```python
from build123d import *

# Parameters (mm, degrees)
BOSS_EXTRUDE1_DEPTH = 160
CUT_EXTRUDE1_START  = -5
SKETCH2_R           = 5
SKETCH2_W           = 10
SKETCH2_H           = 16.92618617
CUT_EXTRUDE1_DEPTH  = 5
CUT_EXTRUDE2_START  = -160
SKETCH2_3_R         = 5
SKETCH2_3_W         = 16.92618617
SKETCH2_3_H         = 10
SKETCH2_3_W_2       = 10
SKETCH2_3_H_2       = 16.92618617
CUT_EXTRUDE2_DEPTH  = 5


with BuildPart() as part:
    # Sketch1 → Boss-Extrude1 (new body)
    with BuildSketch(Plane(origin=(0, 0, 0), x_dir=(1, 0, 0), z_dir=(0, 1, 0))):
        with BuildLine():
            Line((150, 0), (39, 0))
            ThreePointArc((39, 0), (0, -39), (-39, 0))
            Line((-39, 0), (-150, 0))
            ThreePointArc((-150, 0), (0, -150), (150, 0))
        make_face()
    extrude(amount=BOSS_EXTRUDE1_DEPTH)

    # Sketch2 → Cut-Extrude1 (cut)
    with BuildSketch(Plane(origin=(0, 160, 0), x_dir=(1, 0, 0), z_dir=(0, 1, 0)).offset(CUT_EXTRUDE1_START)):
        with BuildLine():
            Line((-52, -5), (-38.678159212, -5))
            ThreePointArc((-38.678159212, -5), (-38.919456633, -2.505173721), (-39, 0))
            Line((-39, 0), (-47, 0))
            ThreePointArc((-47, 0), (-48.464466094, -3.535533906), (-52, -5))
        make_face()
        with BuildLine():
            Line((-47, 0), (-39, 0))
            ThreePointArc((-39, 0), (-38.919456633, 2.505173721), (-38.678159212, 5))
            Line((-38.678159212, 5), (-52, 5))
            ThreePointArc((-52, 5), (-48.464466094, 3.535533906), (-47, 0))
        make_face()
        with BuildLine():
            ThreePointArc((-57, 0), (-55.535533906, -3.535533906), (-52, -5))
            Line((-52, -5), (-52, 0))
            Line((-52, 0), (-57, 0))
        make_face()
        with BuildLine():
            Line((-52, 0), (-52, -5))
            ThreePointArc((-52, -5), (-48.464466094, -3.535533906), (-47, 0))
            Line((-47, 0), (-52, 0))
        make_face()
        with BuildLine():
            Line((-57, 0), (-52, 0))
            Line((-52, 0), (-52, 5))
            ThreePointArc((-52, 5), (-55.535533906, 3.535533906), (-57, 0))
        make_face()
        with BuildLine():
            Line((-52, 5), (-52, 0))
            Line((-52, 0), (-47, 0))
            ThreePointArc((-47, 0), (-48.464466094, 3.535533906), (-52, 5))
        make_face()
        with BuildLine():
            ThreePointArc((38.678159212, 5), (38.919456633, 2.505173721), (39, 0))
            Line((39, 0), (47, 0))
            ThreePointArc((47, 0), (48.464466094, 3.535533906), (52, 5))
            Line((52, 5), (38.678159212, 5))
        make_face()
        with BuildLine():
            ThreePointArc((39, 0), (38.919456633, -2.505173721), (38.678159212, -5))
            Line((38.678159212, -5), (52, -5))
            ThreePointArc((52, -5), (48.464466094, -3.535533906), (47, 0))
            Line((47, 0), (39, 0))
        make_face()
        with BuildLine():
            ThreePointArc((47, 0), (48.464466094, -3.535533906), (52, -5))
            Line((52, -5), (52, 0))
            Line((52, 0), (47, 0))
        make_face()
        with BuildLine():
            Line((52, 0), (52, -5))
            ThreePointArc((52, -5), (55.535533906, -3.535533906), (57, 0))
            Line((57, 0), (52, 0))
        make_face()
        with BuildLine():
            Line((47, 0), (52, 0))
            Line((52, 0), (52, 5))
            ThreePointArc((52, 5), (48.464466094, 3.535533906), (47, 0))
        make_face()
        with BuildLine():
            Line((52, 5), (52, 0))
            Line((52, 0), (57, 0))
            ThreePointArc((57, 0), (55.535533906, 3.535533906), (52, 5))
        make_face()
        with Locations((0, -52)):
            Circle(SKETCH2_R)
        with Locations((0, -43.536906915)):
            Rectangle(SKETCH2_W, SKETCH2_H)
    extrude(amount=CUT_EXTRUDE1_DEPTH, mode=Mode.SUBTRACT)

    # Sketch2_3 → Cut-Extrude2 (cut)
    with BuildSketch(Plane(origin=(0, 160, 0), x_dir=(1, 0, 0), z_dir=(0, 1, 0)).offset(CUT_EXTRUDE2_START)):
        with Locations((0, -52)):
            Circle(SKETCH2_3_R)
        with Locations((-52, 0)):
            Circle(SKETCH2_3_R)
        with Locations((52, 0)):
            Circle(SKETCH2_3_R)
        with Locations((-43.536906915, 0)):
            Rectangle(SKETCH2_3_W, SKETCH2_3_H)
        with Locations((0, -43.536906915)):
            Rectangle(SKETCH2_3_W_2, SKETCH2_3_H_2)
        with Locations((43.536906915, 0)):
            Rectangle(SKETCH2_3_W, SKETCH2_3_H)
    extrude(amount=CUT_EXTRUDE2_DEPTH, mode=Mode.SUBTRACT)


solid = part.part
```
Source: CAD feature listing. Evaluate the final solid. Frame: model axes, mm. A direction names the side the tool comes from. Round coordinates to 2 decimals unless told otherwise and drop trailing zeros. Loops run counter-clockwise (first coordinate to the right, second up) from the corner with the lowest first, then second, coordinate; pieces in that order, holes last.
(1) Pull-direction query (X, two-part tool) for faces 1 (the cylindrical face through (0.86, 78.88, 38.99)), 2 (the flat face through (-2, 160, 74)), 3 (the cylindrical face through (-3.298, 78.88, 149.964)), 4 (the flat face through (0, 155, 48)); classes: +X half, -X half, draft (parallel to the pull), parting line (faces both ways), or undercut.
From the geometry:
face 1: undercut
face 2: draft
face 3: parting line
face 4: undercut
(2) Material intervals for probe 1 along X at (y, z) = (140, 53.5); probe 2 along Z at (x, y) = (-33, 22.5); probe 3 along Z at (x, y) = (71.5, 56), sorted ascending.
From the geometry:
probe 1: x = -140.13 to 140.13
probe 2: z = 20.78 to 146.32
probe 3: z = 0 to 131.86
(3) Contact query for flat-ended pins moving along their axis: pin 1 Ø4 at (y, z) = (156.5, 42.5) entering from +X; pin 2 Ø1.5 at (y, z) = (156.5, 47) entering from -X; pin 3 Ø2.5 at (x, y) = (44.5, 3.5) entering from -Z. Output: stop coordinate, or through.
From the geometry:
pin 1: stops at x = 144.43
pin 2: stops at x = -142.69
pin 3: stops at z = 5
(4) Access query for faces 5 (the flat face through (0, 5, 48)), 6 (the flat face through (-2, 0, 74)). Directions: +Z, -Z, +X, -X, +Y, -Y. A direction counts if a zero-diameter tool reaches every point of the face in a straight line with its end or side. Return the directions, or none.
From the geometry:
face 5: -Z, -Y
face 6: +Z, -Z, +X, -X, -Y
(5) Section query D-D (z = 47.5). Output: boundary loops of the cut face in (x, y), and give its area (3 significant figures).
From the geometry:
outline: (-142.28, 0) - (-5, 0) - (-5, 5) - (5, 5) - (5, 0) - (142.28, 0) - (142.28, 160) - (5, 160) - (5, 155) - (-5, 155) - (-5, 160) - (-142.28, 160) - close
area: 45,400 mm2
(6) Section query B-B (z = 26). Output: boundary loops of the cut face in (x, y).
From the geometry:
outline: (-147.73, 0) - (-29.07, 0) - (-29.07, 160) - (-147.73, 160) - close; (29.07, 0) - (147.73, 0) - (147.73, 160) - (29.07, 160) - close
(7) Section query C-C (y = 145.5). Output: boundary loops of the cut face in (x, z), and give its area (3 significant figures).
From the geometry:
outline: (-150, 0) - (-39, 0) arc R39 cw to (39, 0) - (150, 0) arc R150 ccw to start
area: 33,000 mm2
(8) Section query A-A (x = 0). Output: boundary loops of the cut face in (y, z).
From the geometry:
outline: (0, 57) - (5, 57) - (5, 39) - (155, 39) - (155, 57) - (160, 57) - (160, 150) - (0, 150) - close
